Can you work these out from the model? Positions are in its coordinate system, mm. Face numbers are marked on the shaded views. A direction names the side the tool comes from. Give positions to 0.01 mm unless a question says otherwise; leave off trailing zeros. Order: outer loops, then holes, each group sorted by start corner. A loop starts at its lowest first (then second) coordinate and runs counter-clockwise, first axis right, second up. Notation, with made-up numbers: (66.25, 61) - (74.25, 61) arc R20 cw to (74.25, 100) - close; hole circle Ø1 at (86.25, 7). An arc over 180 degrees is marked (long way). Return JSON: item names as keys, results as strings.
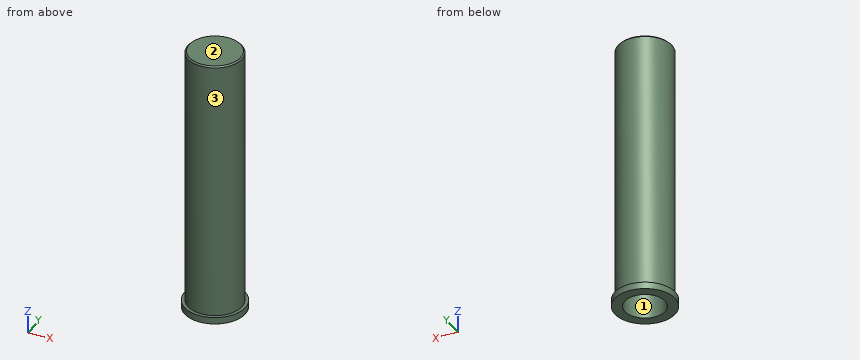
```python
from build123d import *

# Parameters (mm, degrees)
SKETCH_1_R          = 2
EXTRUDE_1_DEPTH     = 20
SKETCH_2_R          = 2.25
EXTRUDE_2_DEPTH     = 0.5
SKETCH_3_R          = 1.5
CUT_EXTRUDE_1_DEPTH = 8
CHAMFER_1_SIZE      = 0.1


with BuildPart() as part:
    # 草图1 → 凸台-拉伸1 (new body)
    with BuildSketch(Plane.XY):
        Circle(SKETCH_1_R)
    extrude(amount=EXTRUDE_1_DEPTH)

    # 草图2 → 凸台-拉伸2 (add)
    with BuildSketch(Plane(origin=(0, 0, 0), x_dir=(-1, 0, 0), z_dir=(0, 0, -1))):
        Circle(SKETCH_2_R)
    extrude(amount=-EXTRUDE_2_DEPTH)

    # 草图3 → 切除-拉伸1 (cut)
    with BuildSketch(Plane(origin=(0, 0, 0), x_dir=(-1, 0, 0), z_dir=(0, 0, -1))):
        Circle(SKETCH_3_R)
    extrude(amount=-CUT_EXTRUDE_1_DEPTH, mode=Mode.SUBTRACT)

    # 倒角1
    chamfer_1_edges = [part.edges().sort_by_distance(p)[0] for p in [
        (-2, 0, 20),
    ]]
    chamfer(chamfer_1_edges, length=CHAMFER_1_SIZE)


solid = part.part
```
1. Suppose I cut it at A-A (y = 0). List the corners of the cut face in (x, z) for me.
Checks:
{"outline": "(-2.25, 0) - (-1.5, 0) - (-1.5, 8) - (1.5, 8) - (1.5, 0) - (2.25, 0) - (2.25, 0.5) - (2, 0.5) - (2, 19.9) - (1.9, 20) - (-1.9, 20) - (-2, 19.9) - (-2, 0.5) - (-2.25, 0.5) - close"}
2. For pin 1 Ø2 at (y, z) = (0.5, 8.5) entering from +X; pin 2 Ø2.5 at (x, y) = (0, 0) entering from -Z; pin 3 Ø1 at (x, z) = (-1, 17) entering from +Y, each with a flat end and sliding along its axis, tell me the tip position at first contact or that it passes through.
Checks:
{"pin 1": "x = 2", "pin 2": "z = 8", "pin 3": "y = 1.94"}
3. Suppose I cut it at C-C (z = 7). List the corners of the cut face in (x, y) for me.
Checks:
{"outline": "circle Ø4 at (0, 0); hole circle Ø3 at (0, 0)"}
4. If I drill on L1, parallel to Y at x = 0, z = 5.5; L2, parallel to Z at x = 1.05, y = 0.85; L3, parallel to Z at x = 2.05, y = -0.1, over which ranges is the centre line in solid material (lowest first)? Write a range as [from, to].
Checks:
{"L1": "[-2, -1.5], [1.5, 2]", "L2": "[8, 20]", "L3": "[0, 0.5]"}
5. On a 3-axis mill with a long thin cutter (end or side, diameter ignored), from which of +Z, -Z, +X, -X, +Y, -Y can I reach the whole of each face in a straight line? I mean the marked faces 1, 2 and 3. Say none if no direction works.
Checks:
{"face 1": "-Z", "face 2": "+Z, +X, -X, +Y, -Y", "face 3": "+Z"}
